Autodesk Inventor part; units mm, degrees
ref_plane "YZ Plane" through (0, 0, 0) normal (1, 0, 0) x (0, 1, 0)
ref_plane "XZ Plane" through (0, 0, 0) normal (0, 1, 0) x (-1, 0, 0)
ref_plane "XY Plane" through (0, 0, 0) normal (0, 0, 1) x (1, 0, 0)
sketch "Boceto1" plane through (0, 0, 0) normal (0, 0, 1) x (1, 0, 0)
  line L0 (-24.5, 24.5) -> (24.5, 24.5)
  line L1 (24.5, 24.5) -> (24.5, -24.5)
  line L2 (24.5, -24.5) -> (-24.5, -24.5)
  line L3 (-24.5, -24.5) -> (-24.5, 24.5)
  line L4 (-24.5, 24.5) -> (24.5, -24.5) construction
  line L5 (24.5, 24.5) -> (-24.5, -24.5) construction
  circle A0 centre (15.5, 15.5) radius 2
  circle A1 centre (-15.5, 15.5) radius 2
  circle A2 centre (-15.5, -15.5) radius 2
  circle A3 centre (15.5, -15.5) radius 2
  circle A4 centre (0, 0) radius 16
  dimension "d0" = 49
  dimension "d1" = 49
  dimension "d2" = 4
  dimension "d3" = 9
  dimension "d6" = 360
  dimension "d10" = 32
extrude "Extrusión1" add sketch "Boceto1" along normal blind 5
properties part number "depth-camera"
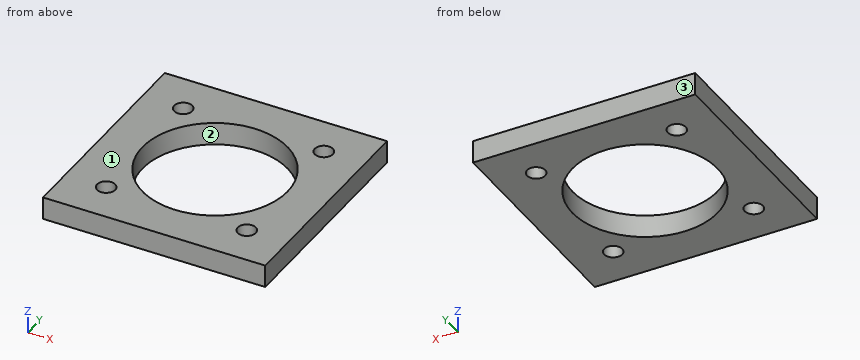
Can you work these out from the model? Positions are in its coordinate system, mm. Face numbers are marked on the shaded views. Round coordinates to 2 decimals unless told otherwise and drop trailing zeros. Order: outer loops, then holes, each group sorted by start corner. A loop starts at its lowest first (then second) coordinate and runs counter-clockwise, first axis right, second up. Notation, with made-up numbers: M 39.5,15.25 L 73.5,15.25 A14 cw 73.5,22.25 Z; hole C 76,2 d11. An arc over 180 degrees is marked long. Use a Markdown table: item, result.
1) Imagine slicing it at A-A (y = 0). List the corners of the cut face in (x, z) for me, then the cut area to 3 significant figures.
Geometry says:
| item | result |
|---|---|
| outline | M -24.5,0 L -16,0 L -16,5 L -24.5,5 Z; M 16,0 L 24.5,0 L 24.5,5 L 16,5 Z |
| area | 85.0 mm² |
2) Imagine slicing it at B-B (z = 2.55). List the corners of the cut face in (x, y) for me.
Geometry says:
| item | result |
|---|---|
| outline | M -24.5,-24.5 L 24.5,-24.5 L 24.5,24.5 L -24.5,24.5 Z; hole C -15.5,-15.5 d4; hole C -15.5,15.5 d4; hole C 0,0 d32; hole C 15.5,-15.5 d4; hole C 15.5,15.5 d4 |
3) If we mould it in two halves opening along Y, with no side actions, what happens to the marked faces 1, 2 and 3? For each: +Y half, -Y half, draft (parallel to the pull), parting line (faces both ways), or undercut.
Geometry says:
| item | result |
|---|---|
| face 1 | draft |
| face 2 | undercut |
| face 3 | +Y half |
4) If I drill on line 1 along X through (y, z) = (17, 1.3); line 2 along Y through (x, z) = (9, 3.65); line 3 along Y through (x, z) = (1.5, 4.45), over which ranges is the centre line in solid material (lowest first)?
Geometry says:
| item | result |
|---|---|
| line 1 | x = -24.5 to -16.82, -14.18 to 14.18, 16.82 to 24.5 |
| line 2 | y = -24.5 to -13.23, 13.23 to 24.5 |
| line 3 | y = -24.5 to -15.93, 15.93 to 24.5 |
